For this review, take the finished solid that the model builds, in its own axes (mm). Round coordinates to 2 decimals unless told otherwise and drop trailing zeros. Order: outer loops, then holes, each group sorted by start corner. A loop starts at its lowest first (then second) coordinate and runs counter-clockwise, first axis right, second up. Notation, with made-up numbers: M 81.5,57.5 L 115.5,57.5 A15 ccw 115.5,72.5 Z; hole C 5.5,55 d10. An arc over 180 degrees is marked long. Answer as a JSON object with one key per item and string values.
from build123d import *

# Parameters (mm, degrees)
SKETCH1_W           = 8
SKETCH1_H           = 8
BOSS_EXTRUDE1_DEPTH = 30
SKETCH2_W           = 8
SKETCH2_H           = 8
BOSS_EXTRUDE2_DEPTH = 10
BOSS_EXTRUDE2_TAPER = 10


with BuildPart() as part:
    # Sketch1 → Boss-Extrude1 (new body)
    with BuildSketch(Plane.XY):
        Rectangle(SKETCH1_W, SKETCH1_H)
    extrude(amount=BOSS_EXTRUDE1_DEPTH)

    # Sketch2 → Boss-Extrude2 (add)
    with BuildSketch(Plane.XY.offset(30)):
        Rectangle(SKETCH2_W, SKETCH2_H)
    extrude(amount=BOSS_EXTRUDE2_DEPTH, taper=BOSS_EXTRUDE2_TAPER)


solid = part.part
1) Add section A-A on x = 1.5. State the section outline as (y, z) points.
Geometry check:
{"outline": "M -4,0 L 4,0 L 4,30 L 2.24,40 L -2.24,40 L -4,30 Z"}
2) Insertion check: P1, Ø1, axis at x = 0, y = -1, coming from the -Z side. The pin has a flat end and moves straight along its axis. Give the tip position at first contact, or say it passes through.
Geometry check:
{"P1": "stops at z = 0"}
3) Add section C-C on z = 33. State the section outline as (x, y) points.
Geometry check:
{"outline": "M -3.47,-3.47 L 3.47,-3.47 L 3.47,3.47 L -3.47,3.47 Z"}
4) For L1, parallel to X at y = 2.25, z = 36; L2, parallel to X at y = -1.75, z = 32.5; L3, parallel to Y at x = -1.75, z = 31, list the stretches that pass through material, from the lowest coordinate up.
Geometry check:
{"L1": "x = -2.94 to 2.94", "L2": "x = -3.56 to 3.56", "L3": "y = -3.82 to 3.82"}
